from build123d import *

# Parameters (mm, degrees)
F0_W     = 82.9564
F0_H     = 25.908
F0_R     = 3.3782
F0_R_2   = 9.779
F1_DEPTH = 6.35
F3_R     = 5.08
F4_SIZE  = 0.508
F2_R     = 0.889
F5_DEPTH = 3.2164930276


with BuildPart() as f1:
    # F0 (on Right) → F1 (new body)
    with BuildSketch(Plane.YZ):
        Rectangle(F0_W, F0_H)
        with Locations((-31.75, 0)):
            Circle(F0_R, mode=Mode.SUBTRACT)
        Circle(F0_R_2, mode=Mode.SUBTRACT)
        with Locations((31.75, 0)):
            Circle(F0_R, mode=Mode.SUBTRACT)
    extrude(amount=F1_DEPTH)

    # F3
    f3_edges = [f1.edges().sort_by_distance(p)[0] for p in [
        (3.175, -41.4782, 12.954),
        (3.175, 41.4782, 12.954),
        (3.175, 41.4782, -12.954),
        (3.175, -41.4782, -12.954),
    ]]
    fillet(f3_edges, radius=F3_R)

    # F4
    f4_edges = [f1.edges().sort_by_distance(p)[0] for p in [
        (0, 28.3718, 0),
        (6.35, 28.3718, 0),
        (0, -35.1282, 0),
        (6.35, -35.1282, 0),
    ]]
    chamfer(f4_edges, length=F4_SIZE)

    # F2 (on face) → F5 (cut, through all)
    with BuildSketch(Plane.XY.offset(12.954)):
        with Locations((3.175, 0)):
            Circle(F2_R)
    extrude(amount=-F5_DEPTH, mode=Mode.SUBTRACT)


solid = f1.part
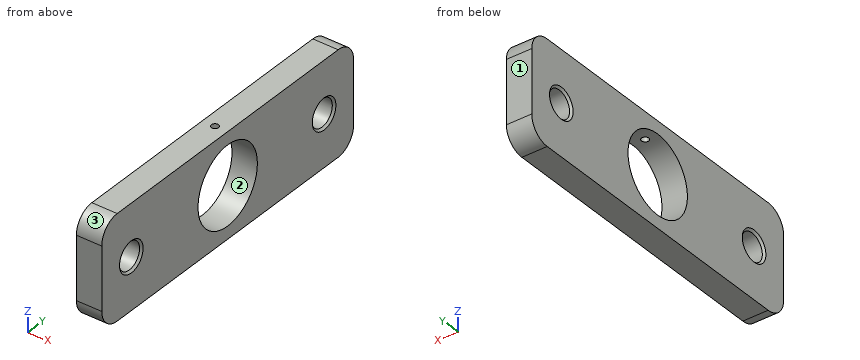
Can you work these out from the model? Positions are in its coordinate system, mm. Face numbers are marked on the shaded views. Coordinates: 2 decimals unless noted, no trailing zeros. Order: outer loops, then holes, each group sorted by start corner. A loop starts at its lowest first (then second) coordinate and runs counter-clockwise, first axis right, second up. Notation, with made-up numbers: (0.25, -32.75) - (44.25, -32.75) arc R21 cw to (44.25, -21.75) - close; hole circle Ø8 at (10.25, 44.25). An arc over 180 degrees is marked (long way). Answer as a JSON object with one key per item and string values. Group by question number.
Q1. Imagine slicing it at D-D (x = 3). Please give me the cut outline in (y, z).
Q2. I need wall thicknesses on line 1 (X direction, y = 0, z = 11.8); line 2 (Z direction, x = 4.25, y = 0); line 3 (Z direction, x = 2.5, y = 31.75). Which ranges of each line are inside material? Lowest first, please. Write a range as from..to.
Q3. Imagine slicing it at C-C (y = 0). Please give me the cut outline in (x, z), and give its area (3 significant figures).
Q4. Imagine slicing it at B-B (z = 0). Please give me the cut outline in (x, y), and give its area (3 significant figures).
Q5. Imagine slicing it at A-A (y = 31.75). Please give me the cut outline in (x, z), and give its area (3 significant figures).
Q6. Will this pin go through, and if not, where does the flat tip stop? P1, Ø2, axis at y = 8.5, z = 0, coming from the +X side.
Q7. We'd pull the mould along Z, two halves only. Please class the marked faces 1, 2 and 3: +Z half, -Z half, draft (parallel to the pull), parting line (faces both ways), or undercut.
Determined:
{
 "1": {"outline": "(-41.48, -7.87) arc R5.08 ccw to (-36.4, -12.95) - (36.4, -12.95) arc R5.08 ccw to (41.48, -7.87) - (41.48, 7.87) arc R5.08 ccw to (36.4, 12.95) - (0.87, 12.95) - (0.87, 9.74) arc R9.78 cw (long way) to (-0.87, 9.74) - (-0.87, 12.95) - (-36.4, 12.95) arc R5.08 ccw to (-41.48, 7.87) - close; hole circle Ø6.76 at (-31.75, 0); hole circle Ø6.76 at (31.75, 0)"},
 "2": {"line 1": "x = 0..2.29, 4.06..6.35", "line 2": "z = -12.95..-9.78, 9.78..12.95", "line 3": "z = -12.95..-3.38, 3.38..12.95"},
 "3": {"outline": "(0, -12.95) - (6.35, -12.95) - (6.35, -9.78) - (0, -9.78) - close; (0, 9.78) - (2.29, 9.78) - (2.29, 12.95) - (0, 12.95) - close; (4.06, 9.78) - (6.35, 9.78) - (6.35, 12.95) - (4.06, 12.95) - close", "area": "34.7 mm2"},
 "4": {"outline": "(0, -41.48) - (6.35, -41.48) - (6.35, -35.64) - (5.84, -35.13) - (0.51, -35.13) - (0, -35.64) - close; (0, -27.86) - (0.51, -28.37) - (5.84, -28.37) - (6.35, -27.86) - (6.35, -9.78) - (0, -9.78) - close; (0, 9.78) - (6.35, 9.78) - (6.35, 27.86) - (5.84, 28.37) - (0.51, 28.37) - (0, 27.86) - close; (0, 35.64) - (0.51, 35.13) - (5.84, 35.13) - (6.35, 35.64) - (6.35, 41.48) - (0, 41.48) - close", "area": "316 mm2"},
 "5": {"outline": "(0, -12.95) - (6.35, -12.95) - (6.35, -3.89) - (5.84, -3.38) - (0.51, -3.38) - (0, -3.89) - close; (0, 3.89) - (0.51, 3.38) - (5.84, 3.38) - (6.35, 3.89) - (6.35, 12.95) - (0, 12.95) - close", "area": "121 mm2"},
 "6": {"P1": "passes through"},
 "7": {"face 1": "draft", "face 2": "undercut", "face 3": "+Z half"}
}
